Can you work these out from the model? Positions are in its coordinate system, mm. A direction names the side the tool comes from. Give positions to 0.01 mm unless a question says otherwise; leave off trailing zeros. Order: outer loops, then holes, each group sorted by start corner. A loop starts at its lowest first (then second) coordinate and runs counter-clockwise, first axis right, second up.
```python
from build123d import *

# Parameters (mm, degrees)
F0_W          = 59.69
F0_H          = 59.69
F1_DEPTH      = 25.4
F1_DEPTH_BACK = 25.4
F3_DEPTH      = 38.1
F4_SIZE       = 6.35
F5_R          = 5.08
F6_R          = 5.08
F7_R          = 2.54
F8_DEPTH      = 25.4
F9_R          = 2.54
F10_DEPTH     = 25.4


# Not quite as in the source:
# - a pattern or mirror of a feature is missing from the dataset's text; its kind, count and spacing are read off the source's solid


with BuildPart() as f1:
    # F0 (on Top) → F1 (new body, two sides)
    with BuildSketch(Plane.XY) as f1_sk:
        Rectangle(F0_W, F0_H)
    extrude(amount=F1_DEPTH)
    extrude(f1_sk.sketch, amount=-F1_DEPTH_BACK)

    # F2 (on face) → F3 (join)
    with BuildSketch(Plane.XY.offset(25.4)):
        Polygon((-23.495, 23.495), (29.845, 23.495), (29.845, 29.845), (-29.845, 29.845), (-29.845, -29.845), (-23.495, -29.845), align=None)
    f3 = extrude(amount=F3_DEPTH)

    # F3_copies: F3 across plane
    add(f3.mirror(Plane(origin=(0, 0, 0), x_dir=(-1, 0, 0), z_dir=(0, 0, -1))))

    # F4
    f4_edges = [f1.edges().sort_by_distance(p)[0] for p in [
        (-26.67, -29.845, 63.5),
        (29.845, 26.67, 63.5),
        (-26.67, -29.845, -63.5),
        (29.845, 26.67, -63.5),
    ]]
    chamfer(f4_edges, length=F4_SIZE)

    # F5
    f5_edges = [f1.edges().sort_by_distance(p)[0] for p in [
        (29.845, -29.845, 0),
    ]]
    fillet(f5_edges, radius=F5_R)

    # F6
    f6_edges = [f1.edges().sort_by_distance(p)[0] for p in [
        (-29.845, 29.845, 0),
    ]]
    fillet(f6_edges, radius=F6_R)

    # F7 (on face) → F8 (cut)
    with BuildSketch(Plane.XZ.offset(-23.495)):
        with Locations((-10.795, 45.72)):
            Circle(F7_R)
        with Locations((14.605, 45.72)):
            Circle(F7_R)
    f8 = extrude(amount=-F8_DEPTH, mode=Mode.SUBTRACT)

    # F8_copies: F8 across plane
    add(f8.mirror(Plane(origin=(0, 0, 0), x_dir=(-1, 0, 0), z_dir=(0, 0, -1))), mode=Mode.SUBTRACT)

    # F9 (on face) → F10 (cut)
    with BuildSketch(Plane.YZ.offset(-23.495)):
        with Locations((-14.605, 45.72)):
            Circle(F9_R)
        with Locations((10.795, 45.72)):
            Circle(F9_R)
    f10 = extrude(amount=-F10_DEPTH, mode=Mode.SUBTRACT)

    # F10_copies: F10 across plane
    add(f10.mirror(Plane(origin=(0, 0, 0), x_dir=(-1, 0, 0), z_dir=(0, 0, -1))), mode=Mode.SUBTRACT)


solid = f1.part
```
1) Suppose I cut it at B-B (y = 20). Please give me the cut outline in (x, z) (3 decimals), and give its area (3 significant figures).
2) Which directions (+Z, -Z, +X, -X, +Y, -Y) give clear straight access to the entire face, cutting with the end or side of a thin tool? Please do faces 1 (the face through (-23.495, -4, 44)), 2 (the face through (-25, 15, -63.5)), 3 (the face through (3, 23.495, -44)).
3) We'd pull the mould along Z, two halves only. Please class faces 4 (the face through (-26.626, -14.936, -48.238)), 5 (the face through (26.714, 26.626, -60.281)), 6 (the face through (-9.43, 26.63, -47.86)), 7 (the face through (-3, -29.845, 1)): +Z half, -Z half, draft (parallel to the pull), parting line (faces both ways), or undercut.
4) Suppose I cut it at C-C (x = -21.5). Please give me the cut outline in (y, z) (3 decimals).
5) Suppose I cut it at D-D (z = -30). Please give me the cut outline in (x, y) (3 decimals), and give its area (3 significant figures).
6) I'm going to push flat-ended pins straight in: pin 1 Ø6 at (y, z) = (-14.605, 45.72) entering from +X (3 decimals); pin 2 Ø19 at (x, z) = (-7, -35) entering from -Y (3 decimals); pin 3 Ø1.5 at (x, y) = (-2, -16.5) entering from +Z; pin 4 Ø4.5 at (x, z) = (-10.795, 45.72) entering from -Y. Where does each tip first touch, or does it pass through?
7) Suppose I cut it at A-A (z = 45.72). Please give me the cut outline in (x, y) (3 decimals).
8) If I drill on line 1 (X direction, y = 28, z = -45.72) (3 decimals); line 2 (Z direction, x = -25, y = 10); line 3 (Z direction, x = 1, y = -9.5), over which ranges is the centre line in solid material (lowest first)?
Results:
1. outline: (-29.845, -63.5) - (-23.495, -63.5) - (-23.495, -25.4) - (29.845, -25.4) - (29.845, 25.4) - (-23.495, 25.4) - (-23.495, 63.5) - (-29.845, 63.5) - close
1. area: 3,520 mm2
2. face 1: +Z, +X, -Y
2. face 2: -Z, +X, -X, +Y, -Y
2. face 3: -Z, +X, -Y
3. face 4: undercut
3. face 5: -Z half
3. face 6: undercut
3. face 7: draft
4. outline: (-29.845, -25.4) - (23.495, -25.4) - (23.495, -63.5) - (29.845, -63.5) - (29.845, 63.5) - (23.495, 63.5) - (23.495, 25.4) - (-29.845, 25.4) - close
5. outline: (-29.845, -29.845) - (-23.495, -29.845) - (-23.495, 23.495) - (29.845, 23.495) - (29.845, 29.845) - (-24.765, 29.845) arc R5.08 ccw to (-29.845, 24.765) - close
5. area: 712 mm2
6. pin 1: stops at x = -23.495
6. pin 2: stops at y = 23.495
6. pin 3: stops at z = 25.4
6. pin 4: passes through
7. outline: (-29.845, -29.845) - (-23.495, -29.845) - (-23.495, -17.145) - (-29.845, -17.145) - close; (-29.845, -12.065) - (-23.495, -12.065) - (-23.495, 8.255) - (-29.845, 8.255) - close; (-29.845, 13.335) - (-23.495, 13.335) - (-23.495, 23.495) - (-13.335, 23.495) - (-13.335, 29.845) - (-24.765, 29.845) arc R5.08 ccw to (-29.845, 24.765) - close; (-8.255, 23.495) - (12.065, 23.495) - (12.065, 29.845) - (-8.255, 29.845) - close; (17.145, 23.495) - (29.845, 23.495) - (29.845, 29.845) - (17.145, 29.845) - close
8. line 1: x = -28.682 to -13.335, -8.255 to 12.065, 17.145 to 29.845
8. line 2: z = -63.5 to -48.13, -43.31 to 43.31, 48.13 to 63.5
8. line 3: z = -25.4 to 25.4
